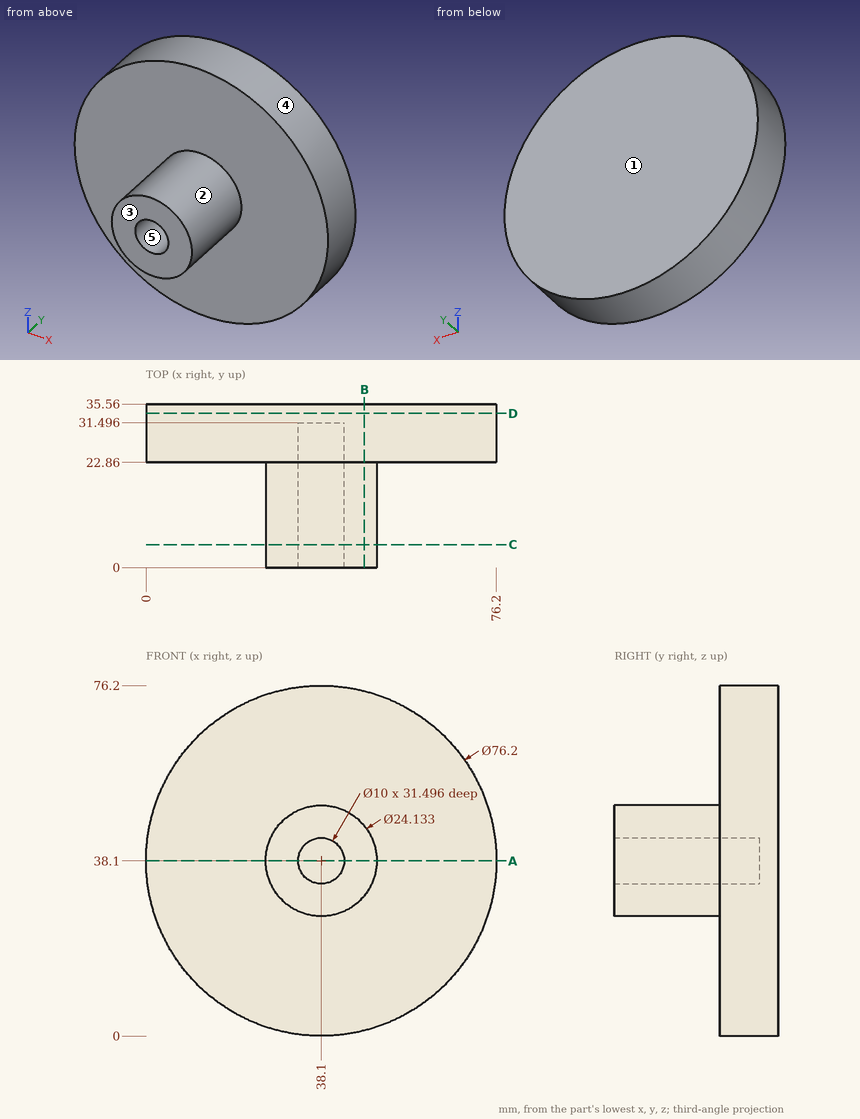
Geometry check sheet. Reference: drawing and pictorial views, mm from the part's lowest x, y, z. A direction names the side the tool comes from. Coordinates: 2 decimals unless noted, no trailing zeros. Order: outer loops, then holes, each group sorted by start corner. A loop starts at its lowest first (then second) coordinate and runs counter-clockwise, first axis right, second up. Notation, with made-up numbers: (17, 76.25) -> (37, 76.25) arc R13 ccw to (37, 96.25) -> close; hole circle Ø2 at (41, 11.5). An arc over 180 degrees is marked (long way). Put each result on its own line as item: value. Start each with the question number.
1) Release check for a two-part mould opening along Z. For the marked faces 3, 4 and 5 record: pulls with the +Z half, pulls with the -Z half, needs draft (parallel to the pull), parting line crosses it, or undercut.
2) Cross-section at C-C (y = 5). Enter the section's corners in (x, z).
3) Cross-section at D-D (y = 33.5). Enter the section's corners in (x, z).
4) Cross-section at A-A (z = 38.1). Enter the section's corners in (x, y).
5) Material ranges on L1, parallel to Z at x = 38, y = 17; L2, parallel to Y at x = 32, z = 15; L3, parallel to Z at x = 40, y = 22.5 (1 decimal), recorded low to high.
6) Cross-section at B-B (x = 47.5). Enter the section's corners in (y, z) (1 decimal).
7) Tool access check on the marked faces 1 and 2. Record the directions out of +Z, -Z, +X, -X, +Y, -Y that give a thin tool (end or side, any length) a straight path to the whole face; none if there is none.
8) Go/stop test with flat-tipped pins: pin 1 (5 mm diameter, centred on x = 38, z = 38, fed in from -Y); pin 2 (10 mm diameter, centred on y = 22, z = 48, fed in from -X); pin 3 (2 mm diameter, centred on x = 52, z = 8, fed in from -Y). Record where each tip stops, or that it passes through.
Geometry check:
1. face 3: needs draft
1. face 4: parting line crosses it
1. face 5: undercut
2. outline: circle Ø24.13 at (38.1, 38.1); hole circle Ø10 at (38.1, 38.1)
3. outline: circle Ø76.2 at (38.1, 38.1)
4. outline: (0, 22.86) -> (26.03, 22.86) -> (26.03, 0) -> (33.1, 0) -> (33.1, 31.5) -> (43.1, 31.5) -> (43.1, 0) -> (50.17, 0) -> (50.17, 22.86) -> (76.2, 22.86) -> (76.2, 35.56) -> (0, 35.56) -> close
5. L1: z = 26.03 to 33.1, 43.1 to 50.17
5. L2: y = 22.86 to 35.56
5. L3: z = 26.2 to 33.5, 42.7 to 50
6. outline: (0, 30.5) -> (22.9, 30.5) -> (22.9, 1.2) -> (35.6, 1.2) -> (35.6, 75) -> (22.9, 75) -> (22.9, 45.7) -> (0, 45.7) -> close
7. face 1: +Z, -Z, +X, -X, +Y
7. face 2: -Y
8. pin 1: stops at y = 31.5
8. pin 2: stops at x = 0.33
8. pin 3: stops at y = 22.86
